Source: three-view drawing plus pictorial views. Frame: mm from the lowest corner of the part. Give positions to 0.01 mm unless a question says otherwise; leave off trailing zeros. Write each loop counter-clockwise with the first axis right and the second up, starting at its lowest first coordinate (ties: lowest second). Pieces come first, ordered by that corner, then holes.
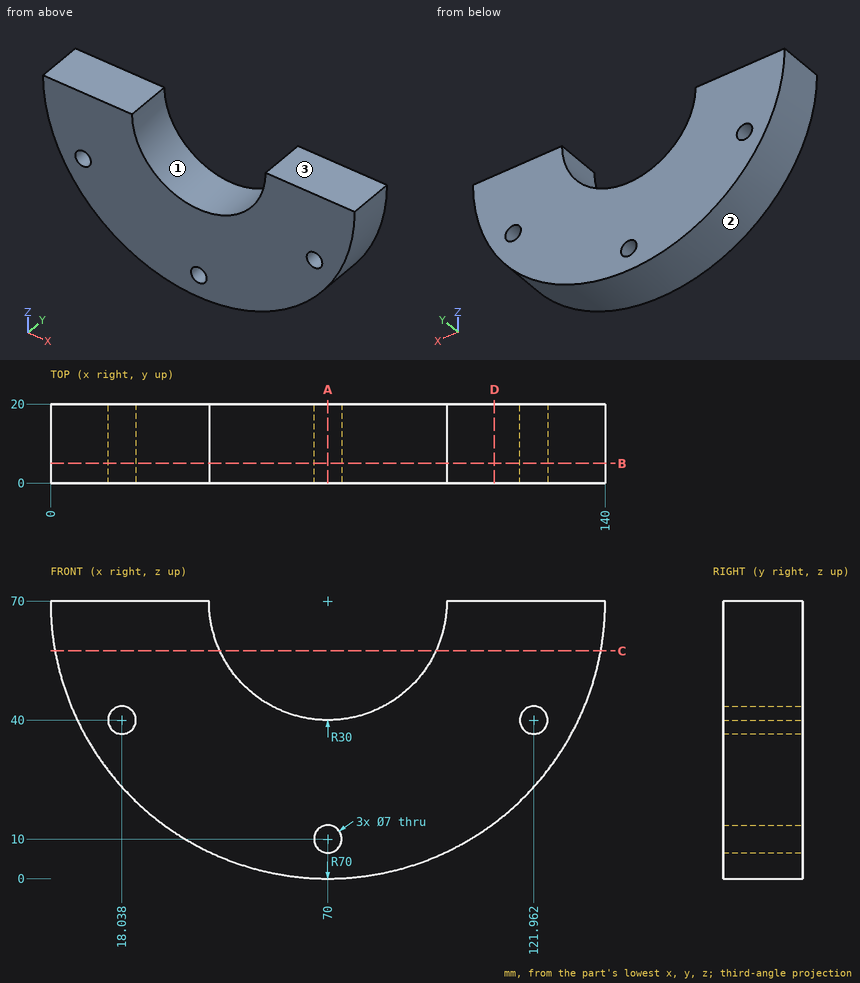
Q1. Ray query, line 1 along Z through (x, y) = (70, 5); line 2 along X through (y, z) = (18.25, 60) (1 decimal); line 3 along Z through (x, y) = (123.5, 5) (1 decimal). Return the intervals inside material, ascending.
Filled sheet:
line 1: z = 0 to 6.5, 13.5 to 40
line 2: x = 0.7 to 41.7, 98.3 to 139.3
line 3: z = 24.9 to 36.9, 43.1 to 70
Q2. Pin query (flat end, axial travel): P1, Ø8, axis at x = 57.5, y = 10.5, coming from the -Z side; P2, Ø6.5, axis at x = 70, z = 10, coming from the -Y side; P3, Ø8, axis at y = 16, z = 43.5, coming from the -X side (1 decimal); P4, Ø1.5, axis at y = 11, z = 10, coming from the -X side (1 decimal). Return the tip coordinate at first contact, or that it passes through.
Filled sheet:
P1: stops at z = 0.52
P2: passes through
P3: stops at x = 3.7
P4: stops at x = 32.7
Q3. Section A-A on x = 70. Output: boundary loops of the cut face in (y, z).
Filled sheet:
outline: (0, 0) - (20, 0) - (20, 6.5) - (0, 6.5) - close; (0, 13.5) - (20, 13.5) - (20, 40) - (0, 40) - close
Q4. Pull-direction query (X, two-part tool) for the marked faces 1, 2 and 3; classes: released by +X, released by -X, zero draft, split by the parting line, or undercut.
Filled sheet:
face 1: undercut
face 2: split by the parting line
face 3: zero draft
Q5. Section D-D on x = 112. Output: boundary loops of the cut face in (y, z), plus the area to 3 significant figures.
Filled sheet:
outline: (0, 14) - (20, 14) - (20, 70) - (0, 70) - close
area: 1,120 mm2
Q6. Section B-B on y = 5. Output: boundary loops of the cut face in (x, z).
Filled sheet:
outline: (0, 70) arc R70 ccw to (140, 70) - (100, 70) arc R30 cw to (40, 70) - close; hole circle Ø7 at (18.04, 40); hole circle Ø7 at (70, 10); hole circle Ø7 at (121.96, 40)
Q7. Section C-C on z = 57.5. Output: boundary loops of the cut face in (x, y) (1 decimal), plus the area to 3 significant figures.
Filled sheet:
outline: (1.1, 0) - (42.7, 0) - (42.7, 20) - (1.1, 20) - close; (97.3, 0) - (138.9, 0) - (138.9, 20) - (97.3, 20) - close
area: 1,660 mm2
